CAD build for the part. Positions are in the model's coordinates, mm. Round coordinates to 2 decimals unless told otherwise and drop trailing zeros. Write each loop counter-clockwise with the first axis right and the second up, starting at its lowest first coordinate (ties: lowest second). Pieces come first, ordered by that corner, then holes. Notation, with made-up numbers: (86, 33) -> (95, 33) arc R22 cw to (95, 51) -> close; hole circle Ø10 at (-23, -9). An arc over 180 degrees is marked (long way). Answer in a Markdown table with one row per item. Add a question column.
```python
from build123d import *

# Parameters (mm, degrees)
F0_R     = 9.5
F1_DEPTH = 1
F2_D     = 3.3
F3_D     = 5
F4_D     = 2.5


with BuildPart() as f1:
    # F0 (on Top) → F1 (new body)
    with BuildSketch(Plane.XY):
        Circle(F0_R)
    extrude(amount=-F1_DEPTH)

    # F2 (through all)
    with Locations(Plane.XY):
        with Locations((0, 6.5), (-6.5, 0), (0, -6.5), (6.5, 0)):
            Hole(F2_D / 2)

    # F3 (through all)
    with Locations(Plane.XY):
        with Locations((-4.2426406871, 4.2426406871)):
            Hole(F3_D / 2)

    # F4 (through all)
    with Locations(Plane.XY):
        with Locations((0, 0)):
            Hole(F4_D / 2)


solid = f1.part
```
Item 1: Saw through at D-D on y = -6.5. Give the cut face in (x, z).
Item 2: Two-plate mould, pull along X, no slides. Class faces 1 (the cylindrical face through (4.38, -8.43, -0.49)), 2 (the flat face through (0, -2, 0)), 3 (the cylindrical face through (8.15, 0.07, -0.51)): +X half, -X half, draft (parallel to the pull), parting line (faces both ways), or undercut.
Item 3: Pin check, flat tips, straight feed: pin 1 (2.5 mm diameter, centred on x = -6.5, y = 0, fed in from -Z); pin 2 (10 mm diameter, centred on x = -4, y = -3, fed in from +Z). Stop position of each tip, or through.
Item 4: Saw through at C-C on x = 0.5. Give the cut face in (y, z), then the cut area to 3 significant figures.
Item 5: Saw through at A-A on y = 0. Give the cut face in (x, z).
Item 6: Saw through at B-B on y = 6.5. Give the cut face in (x, z), then the cut area to 3 significant figures.
Item 7: Drill centre lines: probe 1 along Y at (x, z) = (0, -0.3); probe 2 along Y at (x, z) = (0.5, -0.85); probe 3 along Y at (x, z) = (1.5, -0.6). Where is each one in solid material? Low to high.
Recorded:
| question | item | result |
|---|---|---|
| 1 | outline | (-6.93, -1) -> (-1.65, -1) -> (-1.65, 0) -> (-6.93, 0) -> close; (1.65, -1) -> (6.93, -1) -> (6.93, 0) -> (1.65, 0) -> close |
| 2 | face 1 | parting line |
| 2 | face 2 | draft |
| 2 | face 3 | undercut |
| 3 | pin 1 | through |
| 3 | pin 2 | z = 0 |
| 4 | outline | (-9.49, -1) -> (-8.07, -1) -> (-8.07, 0) -> (-9.49, 0) -> close; (-4.93, -1) -> (-1.15, -1) -> (-1.15, 0) -> (-4.93, 0) -> close; (1.15, -1) -> (4.93, -1) -> (4.93, 0) -> (1.15, 0) -> close; (8.07, -1) -> (9.49, -1) -> (9.49, 0) -> (8.07, 0) -> close |
| 4 | area | 10.4 mm2 |
| 5 | outline | (-9.5, -1) -> (-8.15, -1) -> (-8.15, 0) -> (-9.5, 0) -> close; (-4.85, -1) -> (-1.25, -1) -> (-1.25, 0) -> (-4.85, 0) -> close; (1.25, -1) -> (4.85, -1) -> (4.85, 0) -> (1.25, 0) -> close; (8.15, -1) -> (9.5, -1) -> (9.5, 0) -> (8.15, 0) -> close |
| 6 | outline | (-6.93, -1) -> (-5.32, -1) -> (-5.32, 0) -> (-6.93, 0) -> close; (-3.17, -1) -> (-1.65, -1) -> (-1.65, 0) -> (-3.17, 0) -> close; (1.65, -1) -> (6.93, -1) -> (6.93, 0) -> (1.65, 0) -> close |
| 6 | area | 8.41 mm2 |
| 7 | probe 1 | -9.5 to -8.15, -4.85 to -1.25, 1.25 to 4.85, 8.15 to 9.5 |
| 7 | probe 2 | -9.49 to -8.07, -4.93 to -1.15, 1.15 to 4.93, 8.07 to 9.49 |
| 7 | probe 3 | -9.38 to -7.19, -5.81 to 5.81, 7.19 to 9.38 |
